from build123d import *

# Parameters (mm, degrees)
F0_W     = 777
F0_H     = 474
F1_DEPTH = 12
F2_W     = 6
F2_H     = 474
F3_DEPTH = 6
F4_W     = 6
F4_H     = 474
F5_DEPTH = 6
F6_W     = 765
F6_H     = 6
F7_DEPTH = 6


with BuildPart() as f1:
    # F0 (on Top) → F1 (new body)
    with BuildSketch(Plane.XY):
        with Locations((0, -8.894133)):
            Rectangle(F0_W, F0_H)
    extrude(amount=F1_DEPTH)

    # F2 (on face) → F3 (cut)
    with BuildSketch(Plane(origin=(0, 0, 0), x_dir=(1, 0, 0), z_dir=(0, 0, -1))):
        with Locations((-385.5, 8.894133)):
            Rectangle(F2_W, F2_H)
    extrude(amount=-F3_DEPTH, mode=Mode.SUBTRACT)

    # F4 (on face) → F5 (cut)
    with BuildSketch(Plane(origin=(0, 0, 0), x_dir=(1, 0, 0), z_dir=(0, 0, -1))):
        with Locations((385.5, 8.894133)):
            Rectangle(F4_W, F4_H)
    extrude(amount=-F5_DEPTH, mode=Mode.SUBTRACT)

    # F6 (on face) → F7 (cut)
    with BuildSketch(Plane(origin=(0, 0, 0), x_dir=(1, 0, 0), z_dir=(0, 0, -1))):
        with Locations((0, -225.105867)):
            Rectangle(F6_W, F6_H)
    extrude(amount=-F7_DEPTH, mode=Mode.SUBTRACT)


solid = f1.part
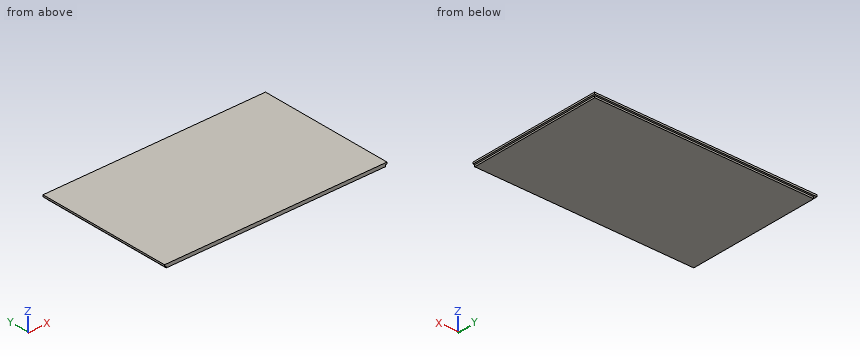
Can you work these out from the model? Positions are in its coordinate system, mm. Round coordinates to 2 decimals unless told otherwise and drop trailing zeros. Write each loop counter-clockwise with the first axis right and the second up, starting at its lowest first coordinate (ties: lowest second). Pieces come first, ordered by that corner, then holes. Notation, with made-up numbers: M 28.5,36.25 L 72.5,36.25 A13 cw 72.5,49.25 Z; hole C -23.75,-6 d2. An arc over 180 degrees is marked long. Use a Markdown table: item, result.
Item 1: I want a section at A-A (z = 3.25). List the corners of the cut face in (x, y) for me, and give its area (3 significant figures).
Found:
| item | result |
|---|---|
| outline | M -382.5,-245.89 L 382.5,-245.89 L 382.5,222.11 L -382.5,222.11 Z |
| area | 358,000 mm2 |
Item 2: If I drill on line 1 along X through (y, z) = (-67, 2.75); line 2 along Y through (x, z) = (-266, 2.25), over which ranges is the centre line in solid material (lowest first)? Write a range as [from, to].
Found:
| item | result |
|---|---|
| line 1 | x = [-382.5, 382.5] |
| line 2 | y = [-245.89, 222.11] |
Item 3: For pin 1 Ø5 at (x, z) = (-114, 3) entering from +Y; pin 2 Ø10 at (x, y) = (-11, -137.5) entering from -Z; pin 3 Ø1.8 at (y, z) = (-33.5, 4) entering from +X; pin 4 Ø3 at (y, z) = (90, 1.5) entering from -X, each with a flat end and sliding along its axis, tell me the tip position at first contact or that it passes through.
Found:
| item | result |
|---|---|
| pin 1 | stops at y = 222.11 |
| pin 2 | stops at z = 0 |
| pin 3 | stops at x = 382.5 |
| pin 4 | stops at x = -382.5 |
